from build123d import *

# Parameters (mm, degrees)
CROQUIS1_R              = 37.5
SALIENTE_EXTRUIR1_DEPTH = 27
CROQUIS2_R              = 31
CORTAR_EXTRUIR1_DEPTH   = 23
CROQUIS3_R              = 22.5
CORTAR_EXTRUIR2_DEPTH   = 23
TALADRO_ROSCADO_M51_D   = 4.2
MATRIZC1_COUNT          = 6


with BuildPart() as part:
    # Croquis1 → Saliente-Extruir1 (new body)
    with BuildSketch(Plane.XY):
        Circle(CROQUIS1_R)
    extrude(amount=SALIENTE_EXTRUIR1_DEPTH)

    # Croquis2 → Cortar-Extruir1 (cut)
    with BuildSketch(Plane.XY.offset(27)):
        Circle(CROQUIS2_R)
    extrude(amount=-CORTAR_EXTRUIR1_DEPTH, mode=Mode.SUBTRACT)

    # Croquis3 → Cortar-Extruir2 (cut)
    with BuildSketch(Plane.XY.offset(4)):
        Circle(CROQUIS3_R)
    extrude(amount=-CORTAR_EXTRUIR2_DEPTH, mode=Mode.SUBTRACT)

    # Taladro roscado M51 (through all)
    with Locations(Plane.XY.offset(27)):
        with Locations((-34.3, 0)):
            taladro_roscado_m51 = Hole(TALADRO_ROSCADO_M51_D / 2)

    # MatrizC1: Taladro roscado M51 ×6 about axis
    matrizc1_axis = Axis((0, 0, 0), (0, 0, 1))
    for i in range(1, MATRIZC1_COUNT):
        add(taladro_roscado_m51.rotate(matrizc1_axis, i * 360 / MATRIZC1_COUNT), mode=Mode.SUBTRACT)


solid = part.part
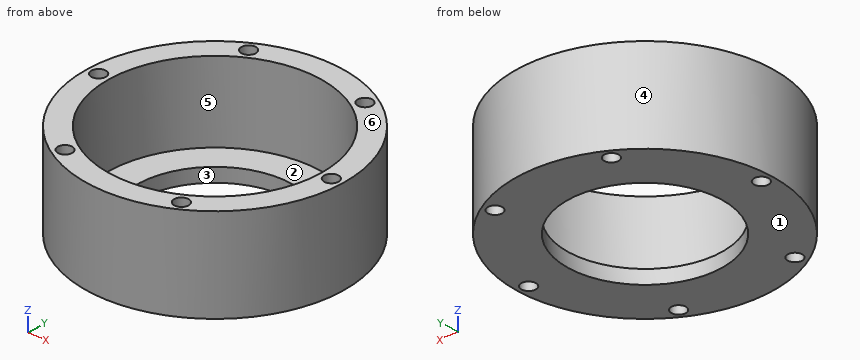
Input: part model. Units: mm. Frame: model coordinates. Face numbers are marked on the shaded views. A direction names the side the tool comes from. Coordinates: 2 decimals unless noted, no trailing zeros. Order: outer loops, then holes, each group sorted by start corner. A loop starts at its lowest first (then second) coordinate and runs counter-clockwise, first axis right, second up.
1. Cut plane A-A, the plane x = 0. Return loops of the section in (y, z), plus the area to 3 significant figures.
Checked values:
outline: (-37.5, 0) - (-22.5, 0) - (-22.5, 4) - (-31, 4) - (-31, 27) - (-37.5, 27) - close; (22.5, 0) - (37.5, 0) - (37.5, 27) - (31, 27) - (31, 4) - (22.5, 4) - close
area: 419 mm2
2. Contact query for flat-ended pins moving along their axis: P1, Ø1.5, axis at x = -25.5, z = 15, coming from the +Y side; P2, Ø2, axis at y = -4, z = 5, coming from the -X side; P3, Ø6, axis at x = 21.5, y = -10.5, coming from the +Z side. Output: stop coordinate, or through.
Checked values:
P1: stops at y = 28.17
P2: stops at x = -37.38
P3: stops at z = 4
3. Cut plane C-C, the plane z = 8. Return loops of the section in (x, y), plus the area to 3 significant figures.
Checked values:
outline: circle Ø75 at (0, 0); hole circle Ø4.2 at (-34.3, 0); hole circle Ø62 at (0, 0); hole circle Ø4.2 at (-17.15, -29.7); hole circle Ø4.2 at (-17.15, 29.7); hole circle Ø4.2 at (17.15, -29.7); hole circle Ø4.2 at (17.15, 29.7); hole circle Ø4.2 at (34.3, 0)
area: 1,320 mm2
4. Draft query along Y for the marked faces 1, 2, 3 and 4. Return one class per face: +Y half, -Y half, draft (parallel to the pull), parting line (faces both ways), or undercut.
Checked values:
face 1: draft
face 2: undercut
face 3: undercut
face 4: parting line
5. Cut plane D-D, the plane x = -17.15. Return loops of the section in (y, z), plus the area to 3 significant figures.
Checked values:
outline: (-33.35, 0) - (-31.8, 0) - (-31.8, 27) - (-33.35, 27) - close; (-27.6, 0) - (-14.56, 0) - (-14.56, 4) - (-25.82, 4) - (-25.82, 27) - (-27.6, 27) - close; (14.56, 0) - (27.6, 0) - (27.6, 27) - (25.82, 27) - (25.82, 4) - (14.56, 4) - close; (31.8, 0) - (33.35, 0) - (33.35, 27) - (31.8, 27) - close
area: 270 mm2
6. Access query for the marked faces 5 and 6. Directions: +Z, -Z, +X, -X, +Y, -Y. A direction counts if a zero-diameter tool reaches every point of the face in a straight line with its end or side. Return the directions, or none.
Checked values:
face 5: +Z
face 6: +Z, +X, -X, +Y, -Y
7. Ray query, line 1 along X through (y, z) = (-1.5, 16); line 2 along Y through (x, z) = (-17.15, 15.25); line 3 along Y through (x, z) = (-15.5, 6.75). Return the intervals inside material, ascending.
Checked values:
line 1: x = -37.47 to -35.77, -32.83 to -30.96, 30.96 to 32.83, 35.77 to 37.47
line 2: y = -33.35 to -31.8, -27.6 to -25.82, 25.82 to 27.6, 31.8 to 33.35
line 3: y = -34.15 to -31, -28.41 to -26.85, 26.85 to 28.41, 31 to 34.15
8. Cut plane B-B, the plane y = 13. Return loops of the section in (x, z).
Checked values:
outline: (-35.17, 0) - (-18.36, 0) - (-18.36, 4) - (-28.14, 4) - (-28.14, 27) - (-35.17, 27) - close; (18.36, 0) - (35.17, 0) - (35.17, 27) - (28.14, 27) - (28.14, 4) - (18.36, 4) - close
